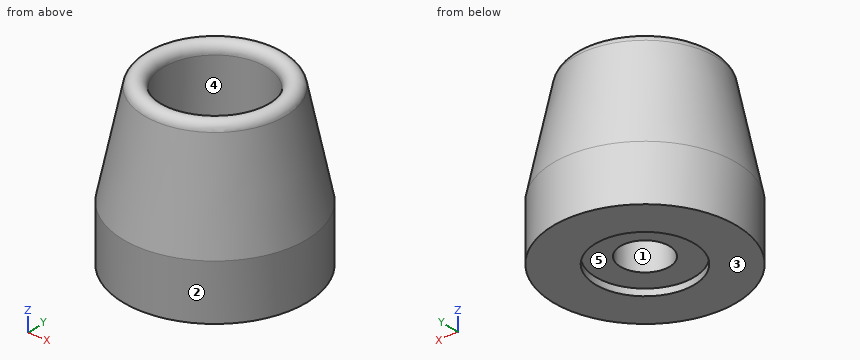
from build123d import *

# Parameters (mm, degrees)
F2_R     = 5.08005
F3_DEPTH = 0.7
F4_R     = 2.532044
F5_DEPTH = 25


with BuildPart() as f1:
    # F0 (on Front) → F1 (revolve)
    with BuildSketch(Plane.XZ):
        with BuildLine():
            Line((-9.45, 0), (0, 0))
            Line((0, 0), (0, 7.03))
            Line((0, 7.03), (-4.8, 7.03))
            ThreePointArc((-4.8, 7.03), (-5.153553, 7.176447), (-5.3, 7.53))
            Line((-5.3, 7.53), (-5.3, 16))
            ThreePointArc((-5.3, 16), (-6.197891, 16.994773), (-7.279148, 16.20315))
            Line((-7.279148, 16.20315), (-9.45, 5.74))
            Line((-9.45, 5.74), (-9.45, 0))
        make_face()
    revolve(axis=Axis((0, 0, 3.515), (0, 0, -1)))

    # F2 (on face) → F3 (cut)
    with BuildSketch(Plane(origin=(0, 0, 0), x_dir=(1, 0, 0), z_dir=(0, 0, -1))):
        Circle(F2_R)
    extrude(amount=-F3_DEPTH, mode=Mode.SUBTRACT)

    # F4 (on face) → F5 (cut)
    with BuildSketch(Plane(origin=(0, 0, 0.7), x_dir=(1, 0, 0), z_dir=(0, 0, -1))):
        Circle(F4_R)
    extrude(amount=-F5_DEPTH, mode=Mode.SUBTRACT)


solid = f1.part
Geometry: final body of the model. Coordinates: model frame, mm. Face numbers are marked on the shaded views. A direction names the side the tool comes from. Round coordinates to 2 decimals unless told otherwise and drop trailing zeros. Write each loop counter-clockwise with the first axis right and the second up, starting at its lowest first coordinate (ties: lowest second). Pieces come first, ordered by that corner, then holes. Notation, with made-up numbers: M -39,73.5 L 4,73.5 A29 ccw 4,98.5 Z; hole C -27.75,46.25 d9. An arc over 180 degrees is marked long. Write item = value, one per line.
Item 1: Section query D-D on z = 11.25. Return loops of the section in (x, y).
Findings:
outline = C 0,0 d16.61; hole C 0,0 d10.6
Item 2: Section query A-A on y = 0. Return loops of the section in (x, z), then the cut area to 3 significant figures.
Findings:
outline = M -9.45,0 L -5.08,0 L -5.08,0.7 L -2.53,0.7 L -2.53,7.03 L -4.8,7.03 A0.5 cw -5.3,7.53 L -5.3,16 A1 ccw -7.28,16.2 L -9.45,5.74 Z; M 2.53,0.7 L 5.08,0.7 L 5.08,0 L 9.45,0 L 9.45,5.74 L 7.28,16.2 A1 ccw 5.3,16 L 5.3,7.53 A0.5 cw 4.8,7.03 L 2.53,7.03 Z
area = 150 mm^2
Item 3: Pull-direction query (Y, two-part tool) for the marked faces 1, 2 and 3; classes: pulls with the +Y half, pulls with the -Y half, needs draft (parallel to the pull), parting line crosses it, or undercut.
Findings:
face_1 = undercut
face_2 = parting line crosses it
face_3 = needs draft
Item 4: Access query for the marked faces 4 and 5. Directions: +Z, -Z, +X, -X, +Y, -Y. A direction counts if a zero-diameter tool reaches every point of the face in a straight line with its end or side. Return the directions, or none.
Findings:
face_4 = +Z
face_5 = -Z
Item 5: Pin query (flat end, axial travel): P1, Ø3, axis at y = -1.5, z = 14.5, coming from the -X side; P2, Ø6, axis at x = -3.5, z = 9.5, coming from the -Y side; P3, Ø6, axis at y = -1.5, z = 8.5, coming from the -X side; P4, Ø6, axis at x = -3, z = 3.5, coming from the +Y side. Return the tip coordinate at first contact, or that it passes through.
Findings:
P1 = -7.87
P2 = -9.01
P3 = -9.44
P4 = 9.45
Item 6: Section query C-C on z = 1.5. Return loops of the section in (x, y), then the cut area to 3 significant figures.
Findings:
outline = C 0,0 d18.9; hole C 0,0 d5.06
area = 260 mm^2
Item 7: Material intervals for line 1 along Y through (x, z) = (0, 3.75); line 2 along X through (y, z) = (-1.5, 10); line 3 along X through (y, z) = (2.5, 15.75), sorted ascending. Write a range as [from, to].
Findings:
line_1 = [-9.45, -2.53], [2.53, 9.45]
line_2 = [-8.43, -5.08], [5.08, 8.43]
line_3 = [-6.94, -4.67], [4.67, 6.94]
